Input: part model. Units: mm. Frame: model coordinates. Coordinates: 2 decimals unless noted, no trailing zeros. Write each loop counter-clockwise with the first axis right and the second up, starting at its lowest first coordinate (ties: lowest second). Pieces come first, ordered by that corner, then holes. Notation, with made-up numbers: M -20.75,54 L 20.25,54 A29 cw 20.25,88 Z; hole C -23,84 d11. An arc over 180 degrees is marked long. Use CSV: the item, a comma, the result in double quotes.
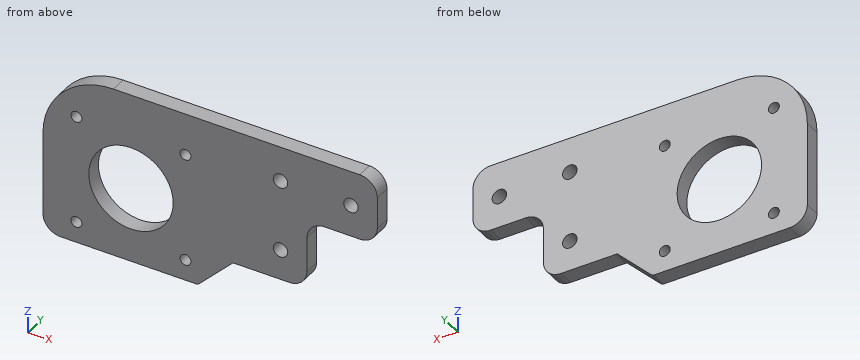
```python
from build123d import *

# Parameters (mm, degrees)
SKETCH1_R           = 2.05
SKETCH1_R_2         = 12
SKETCH1_R_3         = 1.55
BOSS_EXTRUDE1_DEPTH = 4.5
FILLET1_R           = 20
FILLET2_R           = 5
FILLET3_R           = 1


with BuildPart() as part:
    # Sketch1 → Boss-Extrude1 (new body)
    with BuildSketch(Plane(origin=(0, 0, 0), x_dir=(1, 0, 0), z_dir=(0, 1, 0))):
        Polygon((0, 0), (-95, 0), (-95, 49), (-51, 49), (-41, 39), (-20, 39), (-20, 19), (0, 19), align=None)
        with Locations(Location((-7.5, 10, 0), (0, 0, 270))):
            Circle(SKETCH1_R, mode=Mode.SUBTRACT)
        with Locations(Location((-27.5, 10, 0), (0, 0, 270))):
            Circle(SKETCH1_R, mode=Mode.SUBTRACT)
        with Locations(Location((-27.5, 30.337245127, 0), (0, 0, 270))):
            Circle(SKETCH1_R, mode=Mode.SUBTRACT)
        with Locations(Location((-70, 27.5, 0), (0, 0, 270))):
            Circle(SKETCH1_R_2, mode=Mode.SUBTRACT)
        with Locations(Location((-85.5, 43, 0), (0, 0, 270))):
            Circle(SKETCH1_R_3, mode=Mode.SUBTRACT)
        with Locations(Location((-54.5, 43, 0), (0, 0, 270))):
            Circle(SKETCH1_R_3, mode=Mode.SUBTRACT)
        with Locations(Location((-85.5, 12, 0), (0, 0, 270))):
            Circle(SKETCH1_R_3, mode=Mode.SUBTRACT)
        with Locations(Location((-54.5, 12, 0), (0, 0, 270))):
            Circle(SKETCH1_R_3, mode=Mode.SUBTRACT)
    extrude(amount=BOSS_EXTRUDE1_DEPTH)

    # Fillet1
    fillet1_edges = [part.edges().sort_by_distance(p)[0] for p in [
        (-95, 2.25, 0),
    ]]
    fillet(fillet1_edges, radius=FILLET1_R)

    # Fillet2
    fillet2_edges = [part.edges().sort_by_distance(p)[0] for p in [
        (0, 2.25, 0),
        (-95, 2.25, -49),
        (-20, 2.25, -39),
        (-20, 2.25, -19),
        (0, 2.25, -19),
    ]]
    fillet(fillet2_edges, radius=FILLET2_R)

    # Fillet3
    fillet3_edges = [part.edges().sort_by_distance(p)[0] for p in [
        (-51, 2.25, -49),
        (-41, 2.25, -39),
    ]]
    fillet(fillet3_edges, radius=FILLET3_R)


solid = part.part
```
1. Section A-A (z = -43). Return loops of the section in (x, y).
Resolved:
outline,"M -95,0 L -87.05,0 L -87.05,4.5 L -95,4.5 Z; M -83.95,0 L -56.05,0 L -56.05,4.5 L -83.95,4.5 Z; M -52.95,0 L -45,0 L -45,4.5 L -52.95,4.5 Z"
2. Contact query for flat-ended pins moving along their axis: pin 1 Ø8 at (x, z) = (-30.5, -9) entering from -Y; pin 2 Ø2 at (x, y) = (-31.5, 2) entering from -Z. Output: stop coordinate, or through.
Resolved:
pin 1,"stops at y = 0"
pin 2,"stops at z = -39"
3. Section D-D (x = -27.5). Return loops of the section in (y, z).
Resolved:
outline,"M 0,-39 L 4.5,-39 L 4.5,-32.39 L 0,-32.39 Z; M 0,-28.29 L 4.5,-28.29 L 4.5,-12.05 L 0,-12.05 Z; M 0,-7.95 L 4.5,-7.95 L 4.5,0 L 0,0 Z"
4. Section B-B (x = -7.5). Return loops of the section in (y, z).
Resolved:
outline,"M 0,-19 L 4.5,-19 L 4.5,-12.05 L 0,-12.05 Z; M 0,-7.95 L 4.5,-7.95 L 4.5,0 L 0,0 Z"
5. Section C-C (y = 0.9). State how many separate pieces and enclosed holes the cut face has, then the cut area to 3 significant figures.
Resolved:
separate pieces,"1"
enclosed holes,"8"
area,"3,170 mm^2"
6. Material intervals for line 1 (X direction, y = 1, z = -11); line 2 (X direction, y = 2.5, z = -43); line 3 (X direction, y = 1.05, z = -29), sorted ascending. Write a range as [from, to].
Resolved:
line 1,"x = [-92.86, -86.68], [-84.32, -55.68], [-53.32, -29.29], [-25.71, -9.29], [-5.71, 0]"
line 2,"x = [-95, -87.05], [-83.95, -56.05], [-52.95, -45]"
line 3,"x = [-95, -81.91], [-58.09, -29.05], [-25.95, -20]"
